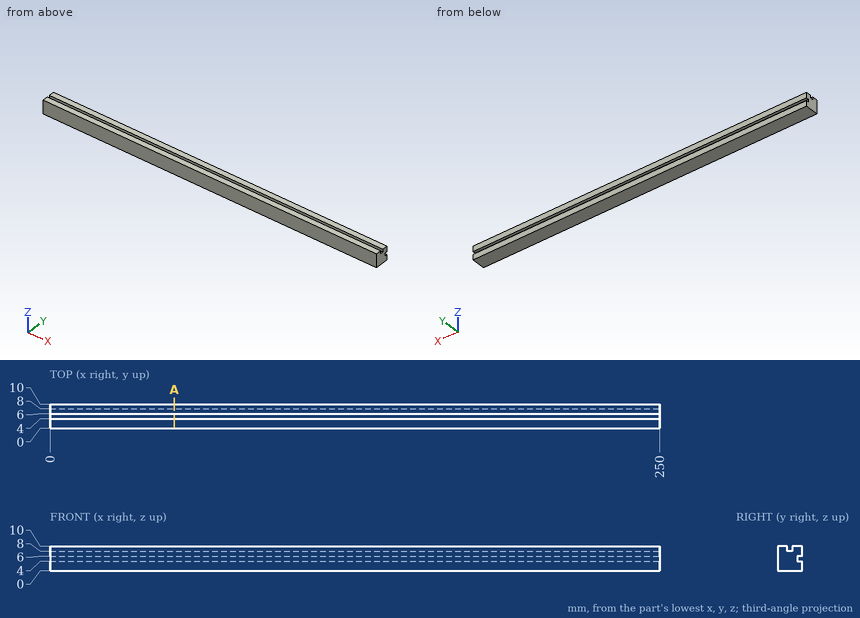
Part print with two shaded views. Sizes in mm from the minimum x, y, z corner. Give positions to 0.01 mm unless a question says otherwise; leave off trailing zeros. Loops run counter-clockwise (first coordinate to the right, second up) from the corner with the lowest first, then second, coordinate; pieces in that order, holes last. Notation, with made-up numbers: (-34.5, -17) - (-30.5, -17) arc R23 ccw to (-30.5, -9) - close; hole circle Ø8 at (-11, 68.5). An arc over 180 degrees is marked (long way). Put each result on its own line as item: value.
Q1. Slice it at A-A (x = 51). Give the cut face in (y, z), plus the area to 3 significant figures.
Filled in:
outline: (0, 0) - (10, 0) - (10, 4) - (8, 4) - (8, 6) - (10, 6) - (10, 10) - (6, 10) - (6, 8) - (4, 8) - (4, 10) - (0, 10) - close
area: 92.0 mm²
Q2. Flat gauge pin, fed straight in: pin 1 (0.6 mm diameter, centred on x = 106, y = 5, fed in from +Z). Where does the tip first touch, or does it go through?
Filled in:
pin 1: stops at z = 8
Q3. Probe line 1 along Z through (x, y) = (209, 8.75); line 2 along Z through (x, y) = (65, 4.25). List the from-to ranges inside material, lowest first.
Filled in:
line 1: z = 0 to 4, 6 to 10
line 2: z = 0 to 8
